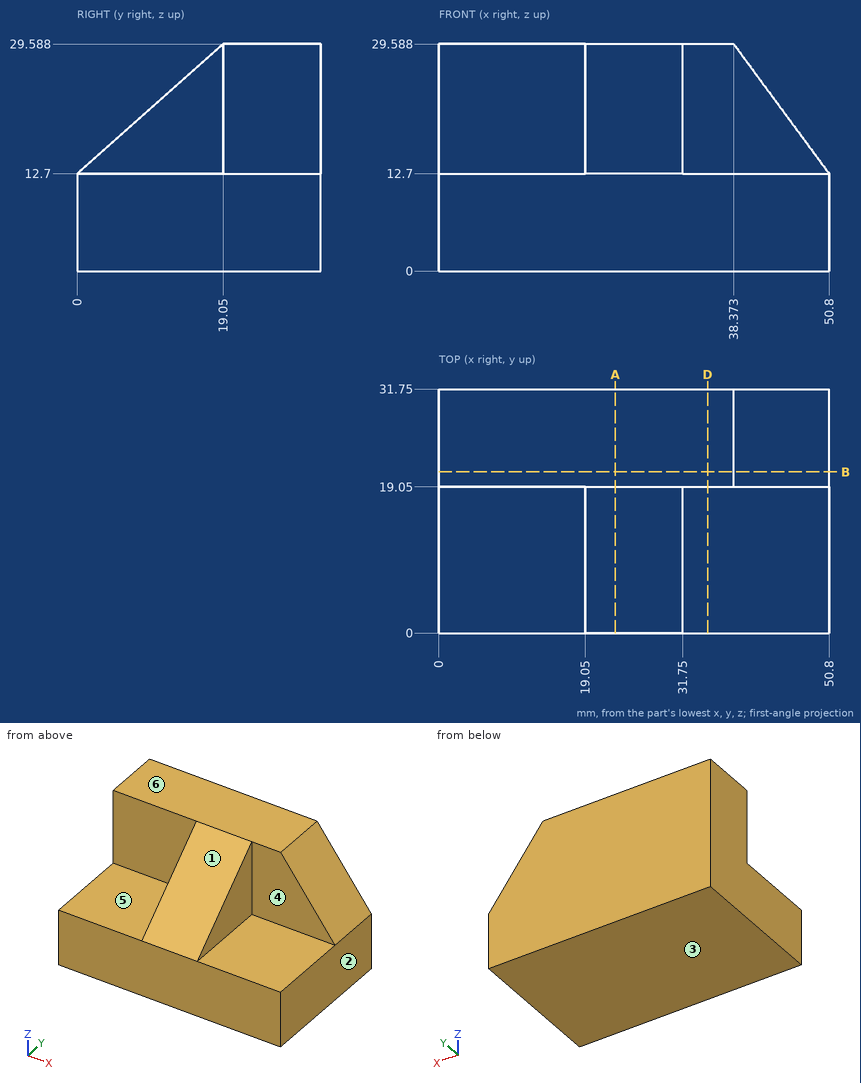
Design review of the part shown in the three views and the two pictorial views. Dimensions are in mm from the part's minimum x, y and z. A direction names the side the tool comes from. Give positions to 0.01 mm unless a question says otherwise; leave off trailing zeros. Loops run counter-clockwise (first coordinate to the right, second up) from the corner with the lowest first, then second, coordinate; pieces in that order, holes last. Notation, with made-up numbers: (59, 30.25) -> (112, 30.25) arc R17 ccw to (112, 59.25) -> close; hole circle Ø2 at (39, -16). An arc over 180 degrees is marked (long way). One line per item, written item: value.
Q1. Draft analysis for pull direction Z (two halves, no side actions). For the marked faces 1, 2 and 3, state which applies: pulls with the +Z half, pulls with the -Z half, needs draft (parallel to the pull), parting line crosses it, or undercut.
Numbers:
face 1: pulls with the +Z half
face 2: needs draft
face 3: pulls with the -Z half
Q2. For L1, parallel to Y at x = 6.5, z = 27.5; L2, parallel to Z at x = 48, y = 8, list the stretches that pass through material, from the lowest coordinate up.
Numbers:
L1: y = 19.05 to 31.75
L2: z = 0 to 12.7
Q3. We need section A-A on x = 23. Give the boundary of the cut face in (y, z).
Numbers:
outline: (0, 0) -> (31.75, 0) -> (31.75, 29.59) -> (19.05, 29.59) -> (0, 12.7) -> close
Q4. We need section B-B on y = 21. Give the boundary of the cut face in (x, z), and give its area (3 significant figures).
Numbers:
outline: (0, 0) -> (50.8, 0) -> (50.8, 12.7) -> (38.37, 29.59) -> (0, 29.59) -> close
area: 1,400 mm^2
Q5. We need section D-D on x = 35. Give the boundary of the cut face in (y, z).
Numbers:
outline: (0, 0) -> (31.75, 0) -> (31.75, 29.59) -> (19.05, 29.59) -> (19.05, 12.7) -> (0, 12.7) -> close
Q6. Machinability: for the marked faces 4, 5 and 6, which of the approach directions +Z, -Z, +X, -X, +Y, -Y give a long, thin tool a straight path to every point of the face, cutting with its end or side? Answer none if there is none.
Numbers:
face 4: +Z, +X, -Y
face 5: +Z, -X, -Y
face 6: +Z, +X, -X, +Y, -Y
Q7. For pin 1 Ø4 at (y, z) = (11, 17) entering from +X; pin 2 Ø5 at (x, z) = (12.5, 17.5) entering from -Y, all flat-tipped, find the tip position at first contact; note any pin that passes through.
Numbers:
pin 1: stops at x = 31.75
pin 2: stops at y = 19.05
